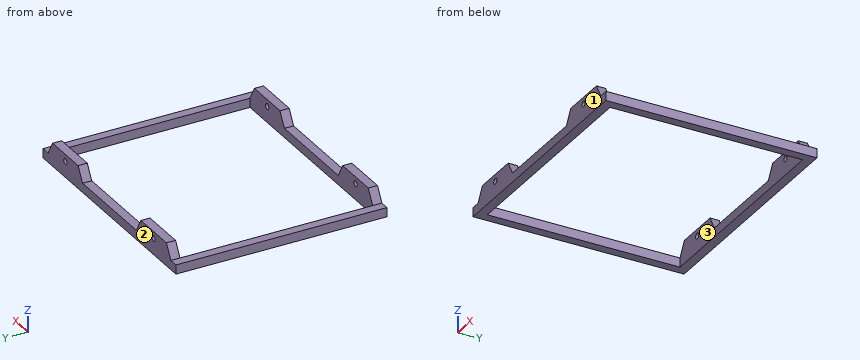
```python
from build123d import *

# Parameters (mm, degrees)
F1_W     = 25.4
F1_H     = 25.4
F4_DEPTH = 25.4
F5_D     = 15.875


with BuildPart() as f2:
    # F2: sweep along a path in F0
    with BuildLine(Plane.XY) as f2_path:
        Line((-304.8, -266.75), (-304.8, 266.75))
        Line((-304.8, 266.75), (304.8, 266.75))
        Line((304.8, 266.75), (304.8, -266.75))
        Line((304.8, -266.75), (-304.8, -266.75))
    # F1 (on Front) → F2 (sweep)
    with BuildSketch(Plane.XZ):
        with Locations((-317.5, 0)):
            Rectangle(F1_W, F1_H)
    sweep(path=f2_path.line, transition=Transition.RIGHT)

    # F3 (on face) → F4 (join, through all)
    with BuildSketch(Plane.XZ.offset(292.15)):
        Polygon((133.8059094878, 12.7), (304.8, 12.7), (282.8029547439, 50.8), (155.8029547439, 50.8), align=None)
    extrude(amount=-F4_DEPTH)

    # F5 (through all)
    with Locations(Plane.XZ.offset(292.15)):
        with Locations((219.3029547439, 31.7)):
            Hole(F5_D / 2)


with BuildPart() as f6_1:
    # F6: instance of F2
    add(f2.part.mirror(Plane.YZ))


with BuildPart() as f2_1:
    add(f2.part)

    add(f6_1.part)  # F7 merges F6_1
    # F7: F6_1, F2 across plane
    add(f6_1.part.mirror(Plane.XZ))
    add(f2.part.mirror(Plane.XZ))


solid = f2_1.part
```
Geometry check sheet. Reference: the model listing, model coordinates, mm. Face numbers are marked on the shaded views. Coordinates: 2 decimals unless noted, no trailing zeros. Loops run counter-clockwise (first coordinate to the right, second up) from the corner with the lowest first, then second, coordinate; pieces in that order, holes last.
Item 1: Release check for a two-part mould opening along Y. For the marked faces 1, 2 and 3 record: released by +Y, released by -Y, zero draft, split by the parting line, or undercut.
Item 2: Sectioned sample at A-A, the plane y = -222.5. Record the boundary of the cut face in (x, z).
Item 3: Go/stop test with a flat-tipped pin: pin 1 Ø20.5 at (x, y) = (-49.5, 277.5) entering from +Z. Record where the tip stops, or that it passes through.
Item 4: Sectioned sample at C-C, the plane z = 31.7. Count the separate pieces of the cut face and the enclosed holes in it, then the cut area to 3 significant figures.
Item 5: Thickness scan on line 1 (X direction, y = -74, z = 12); line 2 (Y direction, x = -176.5, z = 30.5); line 3 (X direction, y = 282, z = 31). Record the ranges inside material, lowest first.
Item 6: Sectioned sample at B-B, the plane x = 83.5. Record the boundary of the cut face in (y, z), then the cut area to 3 significant figures.
Check result:
1. face 1: released by -Y
1. face 2: released by +Y
1. face 3: undercut
2. outline: (-330.2, -12.7) - (-304.8, -12.7) - (-304.8, 12.7) - (-330.2, 12.7) - close; (304.8, -12.7) - (330.2, -12.7) - (330.2, 12.7) - (304.8, 12.7) - close
3. pin 1: stops at z = 12.7
4. separate pieces: 8
4. enclosed holes: 0
4. area: 13,500 mm2
5. line 1: x = -330.2 to -304.8, 304.8 to 330.2
5. line 2: y = -292.15 to -266.75, 266.75 to 292.15
5. line 3: x = -294.23 to -227.21, -211.4 to -144.37, 144.37 to 211.4, 227.21 to 294.23
6. outline: (-292.15, -12.7) - (-266.75, -12.7) - (-266.75, 12.7) - (-292.15, 12.7) - close; (266.75, -12.7) - (292.15, -12.7) - (292.15, 12.7) - (266.75, 12.7) - close
6. area: 1,290 mm2
